```python
from build123d import *

# Parameters (mm, degrees)
BOSS_EXTRUDE1_DEPTH = 20
FILLET1_R           = 0.5


with BuildPart() as part:
    # Sketch1 → Boss-Extrude1 (new body)
    with BuildSketch(Plane(origin=(0, 0, 0), x_dir=(0, 0, -1), z_dir=(1, 0, 0))):
        with BuildLine():
            Line((3.25, -1.870828693), (3.25, 1.870828693))
            ThreePointArc((3.25, 1.870828693), (-3.75, 0), (3.25, -1.870828693))
        make_face()
    extrude(amount=BOSS_EXTRUDE1_DEPTH)

    # Fillet1
    fillet1_edges = [part.edges().sort_by_distance(p)[0] for p in [
        (0, 0, 3.75),
        (0, 0, -3.25),
        (20, 0, -3.25),
        (10, -1.870828693, -3.25),
        (10, 1.870828693, -3.25),
        (20, 0, 3.75),
    ]]
    fillet(fillet1_edges, radius=FILLET1_R)


solid = part.part
```
Input: part model. Units: mm. Frame: model coordinates. Round coordinates to 2 decimals unless told otherwise and drop trailing zeros. Loops run counter-clockwise (first coordinate to the right, second up) from the corner with the lowest first, then second, coordinate; pieces in that order, holes last. Notation, with made-up numbers: M 73,45.25 L 112,45.25 A24 cw 112,81.25 Z; hole C 58,-40 d9. An arc over 180 degrees is marked long. Answer in a Markdown table with one row per item. Add a question column.
1. Section A-A (x = 8). Output: boundary loops of the cut face in (y, z).
2. Ray query, probe 1 along Y at (x, z) = (16, -2); probe 2 along Y at (x, z) = (8.5, -1.75); probe 3 along Z at (x, y) = (14.25, -0.75). Return the intervals inside material, ascending.
3. Contact query for a flat-ended pin moving along its axis: pin 1 (1 mm diameter, centred on x = 2.5, z = 2, fed in from -Y). Output: stop coordinate, or through.
Values follow:
| question | item | result |
|---|---|---|
| 1 | outline | M -2,-3.17 A0.5 ccw -1.73,-3.25 L 1.73,-3.25 A0.5 ccw 2,-3.17 A3.75 ccw long Z |
| 2 | probe 1 | -3.17 to 3.17 |
| 2 | probe 2 | -3.32 to 3.32 |
| 2 | probe 3 | -3.25 to 3.67 |
| 3 | pin 1 | y = -3.44 |
